Read the model definition and answer for the solid it produces. Units are mm, in the model's axes. A direction names the side the tool comes from. Coordinates: 2 decimals unless noted, no trailing zeros. Order: outer loops, then holes, each group sorted by start corner. A loop starts at its lowest first (then second) coordinate and runs counter-clockwise, first axis right, second up. Notation, with made-up numbers: (-40, 1.5) -> (-25, 1.5) arc R12 cw to (-25, 14.5) -> close; hole circle Ø6 at (-34.5, 87.5). An arc over 180 degrees is marked (long way). Answer in a Markdown table with one row per item.
from build123d import *

# Parameters (mm, degrees)
EXTRUDE_1_DEPTH          = 5
SKETCH_3_R               = 22
CUT_EXTRUDE_1_DEPTH      = 75.79973262
SKETCH_4_R               = 1.6
CUT_EXTRUDE_3_DEPTH      = 75.79973262
SKETCH_9_R               = 1.6
SKETCH_9_R_2             = 22
EXTRUDE_2_DEPTH          = 2
FILLET_1_R               = 1
CUT_EXTRUDE_4_DEPTH      = 68.779052811
CUT_EXTRUDE_4_DEPTH_BACK = 68.779052811


with BuildPart() as part:
    # Эскиз2 → Бобышка-Вытянуть1 (new body)
    with BuildSketch(Plane(origin=(0, -5, 0), x_dir=(-1, 0, 0), z_dir=(0, -1, 0))):
        with BuildLine():
            Line((-28.05572809, -61), (-3.94427191, -61))
            ThreePointArc((-3.94427191, -61), (-2.610938577, -60.490711985), (-1.95665593, -59.222222222))
            ThreePointArc((-1.95665593, -59.222222222), (0.333333333, -54.782508053), (5, -53))
            Line((5, -53), (9, -53))
            ThreePointArc((9, -53), (10.414213562, -52.414213562), (11, -51))
            Line((11, -51), (11, -9.854480973))
            ThreePointArc((11, -9.854480973), (10.513111175, -8.546622199), (9.289505428, -7.875545247))
            ThreePointArc((9.289505428, -7.875545247), (6.355962769, -7.049175653), (3.731345838, -5.5))
            Line((3.731345838, -5.5), (-35.731345838, -5.5))
            ThreePointArc((-35.731345838, -5.5), (-38.355962769, -7.049175653), (-41.289505428, -7.875545247))
            ThreePointArc((-41.289505428, -7.875545247), (-42.513111175, -8.546622199), (-43, -9.854480973))
            Line((-43, -9.854480973), (-43, -51))
            ThreePointArc((-43, -51), (-42.414213562, -52.414213562), (-41, -53))
            Line((-41, -53), (-37, -53))
            ThreePointArc((-37, -53), (-32.333333333, -54.782508053), (-30.04334407, -59.222222222))
            ThreePointArc((-30.04334407, -59.222222222), (-29.389061423, -60.490711985), (-28.05572809, -61))
        make_face()
    extrude(amount=EXTRUDE_1_DEPTH)

    # Эскиз3 → Вырез-Вытянуть1 (cut, through all)
    with BuildSketch(Plane.XZ.offset(10)):
        with Locations(Location((16, 34.5, 0), (0, 0, 270))):
            Circle(SKETCH_3_R)
    extrude(amount=-CUT_EXTRUDE_1_DEPTH, mode=Mode.SUBTRACT)

    # Эскиз4 → Вырез-Вытянуть3 (cut, through all)
    with BuildSketch(Plane.XZ.offset(10)):
        with Locations(Location((38.5, 20, 0), (0, 0, 270))):
            Circle(SKETCH_4_R)
        with Locations(Location((-6.5, 20, 0), (0, 0, 270))):
            Circle(SKETCH_4_R)
        with Locations(Location((-6.5, 46, 0), (0, 0, 270))):
            Circle(SKETCH_4_R)
        with Locations(Location((38.5, 46, 0), (0, 0, 270))):
            Circle(SKETCH_4_R)
        with Locations(Location((24, 57, 0), (0, 0, 270))):
            Circle(SKETCH_4_R)
        with Locations(Location((8, 57, 0), (0, 0, 270))):
            Circle(SKETCH_4_R)
        with Locations(Location((16, 9, 0), (0, 0, 270))):
            Circle(SKETCH_4_R)
    extrude(amount=-CUT_EXTRUDE_3_DEPTH, mode=Mode.SUBTRACT)

    # Эскиз9 → Бобышка-Вытянуть2 (add)
    with BuildSketch(Plane.XZ.offset(10)):
        with BuildLine():
            Line((28.05572809, 61), (3.94427191, 61))
            ThreePointArc((3.94427191, 61), (2.610938577, 60.490711985), (1.95665593, 59.222222222))
            ThreePointArc((1.95665593, 59.222222222), (-0.333333333, 54.782508053), (-5, 53))
            Line((-5, 53), (-9, 53))
            ThreePointArc((-9, 53), (-10.414213562, 52.414213562), (-11, 51))
            Line((-11, 51), (-11, 9.854480973))
            ThreePointArc((-11, 9.854480973), (-10.513111175, 8.546622199), (-9.289505428, 7.875545247))
            ThreePointArc((-9.289505428, 7.875545247), (-6.355962769, 7.049175653), (-3.731345838, 5.5))
            Line((-3.731345838, 5.5), (35.731345838, 5.5))
            ThreePointArc((35.731345838, 5.5), (38.355962769, 7.049175653), (41.289505428, 7.875545247))
            ThreePointArc((41.289505428, 7.875545247), (42.513111175, 8.546622199), (43, 9.854480973))
            Line((43, 9.854480973), (43, 51))
            ThreePointArc((43, 51), (42.414213562, 52.414213562), (41, 53))
            Line((41, 53), (37, 53))
            ThreePointArc((37, 53), (32.333333333, 54.782508053), (30.04334407, 59.222222222))
            ThreePointArc((30.04334407, 59.222222222), (29.389061423, 60.490711985), (28.05572809, 61))
        make_face()
        with Locations(Location((38.5, 46, 0), (0, 0, 270))):
            Circle(SKETCH_9_R, mode=Mode.SUBTRACT)
        with Locations(Location((24, 57, 0), (0, 0, 270))):
            Circle(SKETCH_9_R, mode=Mode.SUBTRACT)
        with Locations(Location((38.5, 20, 0), (0, 0, 270))):
            Circle(SKETCH_9_R, mode=Mode.SUBTRACT)
        with Locations(Location((16, 9, 0), (0, 0, 270))):
            Circle(SKETCH_9_R, mode=Mode.SUBTRACT)
        with Locations(Location((-6.5, 20, 0), (0, 0, 270))):
            Circle(SKETCH_9_R, mode=Mode.SUBTRACT)
        with Locations(Location((-6.5, 46, 0), (0, 0, 270))):
            Circle(SKETCH_9_R, mode=Mode.SUBTRACT)
        with Locations(Location((8, 57, 0), (0, 0, 270))):
            Circle(SKETCH_9_R, mode=Mode.SUBTRACT)
        with Locations(Location((16, 34.5, 0), (0, 0, 270))):
            Circle(SKETCH_9_R_2, mode=Mode.SUBTRACT)
    extrude(amount=EXTRUDE_2_DEPTH)

    # Скругление1
    # the kernel refuses this fillet: 1 mm, written as the material it takes off along each edge
    with BuildSketch(Plane(origin=(16, -5, 34.5), x_dir=(0, 0, -1), z_dir=(-1, 0, 0))) as fillet_1_piece_1:
        with BuildLine():
            CenterArc((22 + FILLET_1_R, FILLET_1_R), FILLET_1_R, 180, 90)
            Line((22, FILLET_1_R), (22, 0))
            Line((22, 0), (22 + FILLET_1_R, 0))
        make_face()
    revolve(axis=Axis((16, -5, 34.5), (0, -1, 0)), mode=Mode.SUBTRACT)

    # Эскиз12 → Вырез-Вытянуть4 (cut, two sides: drawn at the far end of the back side and taken through both)
    with BuildSketch(Plane(origin=(16, 0, 0), x_dir=(0, 0, 1), z_dir=(1, 0, 0)).offset(-CUT_EXTRUDE_4_DEPTH_BACK)):
        Polygon((61, 12), (61, 6), (59.3, 12), align=None)
    extrude(amount=CUT_EXTRUDE_4_DEPTH + CUT_EXTRUDE_4_DEPTH_BACK, mode=Mode.SUBTRACT)


solid = part.part
Q1. The part is cut by section B-B (y = -9.25). Give the number of separate pieces and of enclosed holes in the cut face, then the cut area to 3 significant figures.
Outcome:
| item | result |
|---|---|
| separate pieces | 1 |
| enclosed holes | 8 |
| area | 1,180 mm² |
Q2. The part is cut by section A-A (x = 16). Write down the section's boundary in (y, z).
Outcome:
| item | result |
|---|---|
| outline | (-12, 5.5) -> (-5, 5.5) -> (-5, 7.4) -> (-12, 7.4) -> close; (-12, 10.6) -> (-5, 10.6) -> (-5, 11.5) arc R1 ccw to (-6, 12.5) -> (-12, 12.5) -> close; (-12, 56.5) -> (-6, 56.5) arc R1 ccw to (-5, 57.5) -> (-5, 61) -> (-6, 61) -> (-12, 59.3) -> close |
Q3. Consider line 1 (Z direction, x = 9, y = -9.75); line 2 (X direction, y = -10.85, z = 46) (3 decimals); line 3 (Z direction, x = 25, y = -6). Determine where each line is inside the solid, lowest interval first.
Outcome:
| item | result |
|---|---|
| line 1 | 5.5 to 13.64, 55.36 to 55.75, 58.25 to 59.94 |
| line 2 | -11 to -8.1, -4.9 to -2.755, 34.755 to 36.9, 40.1 to 43 |
| line 3 | 5.5 to 14.43, 54.57 to 55.75, 58.25 to 61 |
Q4. Given pin 1 (1.9 mm diameter, centred on x = 16, z = 9, fed in from +Y); pin 2 (3 mm diameter, centred on x = 39, y = -8.5, fed in from +Z), each flat-ended and moving along its own axis, determine where each tip first touches the part or whether it passes through.
Outcome:
| item | result |
|---|---|
| pin 1 | through |
| pin 2 | z = 53 |
Q5. The part is cut by section C-C (z = 9). Write down the section's boundary in (x, y).
Outcome:
| item | result |
|---|---|
| outline | (-10.81, -12) -> (14.4, -12) -> (14.4, -5) -> (-10.81, -5) -> close; (17.6, -12) -> (42.81, -12) -> (42.81, -5) -> (17.6, -5) -> close |
Q6. For faces 1 (the face through (4, -12, 15)), 2 (the face through (-7, -8, 53)), 3 (the face through (39, -8, 53)), determine the directions among +Z, -Z, +X, -X, +Y, -Y from which every point of the face is accessible in a straight line to the end or side of a thin tool.
Outcome:
| item | result |
|---|---|
| face 1 | +Z, -Z, +X, -X, -Y |
| face 2 | +Z, -X, +Y, -Y |
| face 3 | +Z, +X, +Y, -Y |
